from build123d import *
from build123d.topology import SkipClean

# Parameters (mm, degrees)
BOSS_EXTRUDE1_DEPTH      = 3.81
BOSS_EXTRUDE1_DEPTH_BACK = 6.35
SKETCH1_R                = 49.4538
SKETCH2_R                = 49.4538
BOSS_EXTRUDE2_DEPTH      = 381
SHELL1_T                 = -3.175
CUT_EXTRUDE1_DEPTH       = 398.363186857
BOSS_EXTRUDE3_DEPTH      = 3.81
SKETCH7_R                = 49.4538
SKETCH7_R_2              = 45.085
CUT_EXTRUDE2_DEPTH       = 6.35
BOSS_EXTRUDE4_START      = 7.62
BOSS_EXTRUDE4_DEPTH      = 7.62
SKETCH10_R               = 35.56
CUT_EXTRUDE3_DEPTH       = 6.35
SKETCH11_R               = 8.382
CUT_EXTRUDE4_DEPTH       = 5.08
SKETCH12_R               = 6.0325
CUT_EXTRUDE5_DEPTH       = 402.739558289
BOSS_EXTRUDE5_DEPTH      = 5.08
SKETCH14_R               = 4.191
CUT_EXTRUDE6_DEPTH       = 405.866453376
BOSS_EXTRUDE6_START      = 6.35
SKETCH15_R               = 4.191
SKETCH15_R_2             = 6.0325
BOSS_EXTRUDE6_DEPTH      = 6.35


with BuildPart() as part:
    # Sketch1 → Boss-Extrude1 (new, two sides: drawn at the far end of the back side and taken through both)
    with BuildSketch(Plane(origin=(0, 0, 0), x_dir=(1, 0, 0), z_dir=(0, 1, 0)).offset(-BOSS_EXTRUDE1_DEPTH_BACK)):
        with Locations(Location((0, 0, 0), (0, 0, 270))):
            Circle(SKETCH1_R)
    extrude(amount=BOSS_EXTRUDE1_DEPTH + BOSS_EXTRUDE1_DEPTH_BACK)

    # Sketch2 → Boss-Extrude2 (add)
    with BuildSketch(Plane(origin=(0, 3.81, 0), x_dir=(1, 0, 0), z_dir=(0, 1, 0))):
        with Locations(Location((0, 0, 0), (0, 0, 270))):
            Circle(SKETCH2_R)
    extrude(amount=BOSS_EXTRUDE2_DEPTH)

    # Shell1
    shell1_openings = [part.faces().sort_by_distance(p)[0] for p in [
        (0, 384.81, 0),
    ]]
    offset(amount=SHELL1_T, openings=shell1_openings, kind=Kind.INTERSECTION)

    # Sketch4 → Cut-Extrude1 (cut, through all)
    with BuildSketch(Plane.XZ.offset(6.35)):
        with BuildLine():
            Line((49.4538, 0), (12.7, 0))
            ThreePointArc((12.7, 0), (0, -12.7), (-12.7, 0))
            Line((-12.7, 0), (-49.4538, 0))
            ThreePointArc((-49.4538, 0), (0, -49.4538), (49.4538, 0))
        make_face()
    extrude(amount=-CUT_EXTRUDE1_DEPTH, mode=Mode.SUBTRACT)

    # Sketch5 → Boss-Extrude3 (add)
    with BuildSketch(Plane(origin=(0, -3.175, 0), x_dir=(1, 0, 0), z_dir=(0, 1, 0))):
        with BuildLine():
            Line((-46.2788, 0), (-12.7, 0))
            ThreePointArc((-12.7, 0), (0, 12.7), (12.7, 0))
            Line((12.7, 0), (46.2788, 0))
            ThreePointArc((46.2788, 0), (0, -46.2788), (-46.2788, 0))
        make_face()
    extrude(amount=BOSS_EXTRUDE3_DEPTH)

    # Sketch7 → Cut-Extrude2 (cut)
    with BuildSketch(Plane.XZ.offset(6.35)):
        Circle(SKETCH7_R)
        Circle(SKETCH7_R_2, mode=Mode.SUBTRACT)
    extrude(amount=-CUT_EXTRUDE2_DEPTH, mode=Mode.SUBTRACT)

    # Sketch9 → Boss-Extrude4 (add)
    with SkipClean():  # the faces are left unmerged after this step: merging them gives an invalid solid
        with BuildSketch(Plane.XZ.offset(6.35).offset(BOSS_EXTRUDE4_START)):
            with BuildLine():
                Line((45.085, 0), (12.7, 0))
                ThreePointArc((12.7, 0), (0, -12.7), (-12.7, 0))
                Line((-12.7, 0), (-45.085, 0))
                ThreePointArc((-45.085, 0), (0, 45.085), (45.085, 0))
            make_face()
        extrude(amount=-BOSS_EXTRUDE4_DEPTH)
    add(part.part.scale(1), mode=Mode.REPLACE)  # the faces are merged on a copy

    # Sketch10 → Cut-Extrude3 (cut)
    with BuildSketch(Plane(origin=(0, 0.635, 0), x_dir=(1, 0, 0), z_dir=(0, 1, 0))):
        Circle(SKETCH10_R)
    extrude(amount=-CUT_EXTRUDE3_DEPTH, mode=Mode.SUBTRACT)

    # Sketch11 → Cut-Extrude4 (cut)
    with BuildSketch(Plane(origin=(0, -5.715, 0), x_dir=(1, 0, 0), z_dir=(0, 1, 0))):
        with Locations(Location((0, 0, 0), (0, 0, 270))):
            Circle(SKETCH11_R)
    cut_extrude4 = extrude(amount=-CUT_EXTRUDE4_DEPTH, mode=Mode.SUBTRACT)

    # Sketch12 → Cut-Extrude5 (cut, through all)
    with BuildSketch(Plane(origin=(0, -10.795, 0), x_dir=(1, 0, 0), z_dir=(0, 1, 0))):
        with Locations(Location((0, 0, 0), (0, 0, 270))):
            Circle(SKETCH12_R)
    extrude(amount=-CUT_EXTRUDE5_DEPTH, mode=Mode.SUBTRACT)

    # Sketch13 → Boss-Extrude5 (add)
    with SkipClean():  # the faces are left unmerged after this step: merging them gives an invalid solid
        with BuildSketch(Plane(origin=(0, 0.635, 0), x_dir=(1, 0, 0), z_dir=(0, 1, 0))):
            with BuildLine():
                Line((-46.2788, 0), (-35.56, 0))
                ThreePointArc((-35.56, 0), (0, -35.56), (35.56, 0))
                Line((35.56, 0), (46.2788, 0))
                ThreePointArc((46.2788, 0), (0, -46.2788), (-46.2788, 0))
            make_face()
        extrude(amount=BOSS_EXTRUDE5_DEPTH)
    add(part.part.scale(1), mode=Mode.REPLACE)  # the faces are merged on a copy

    # Sketch14 → Cut-Extrude6 (cut, through all)
    with BuildSketch(Plane.XZ.offset(13.97)):
        with Locations(Location((0, 15.24, 0), (0, 0, 270))):
            Circle(SKETCH14_R)
    extrude(amount=-CUT_EXTRUDE6_DEPTH, mode=Mode.SUBTRACT)

    # Sketch15 → Boss-Extrude6 (add)
    with BuildSketch(Plane.XZ.offset(13.97).offset(BOSS_EXTRUDE6_START)):
        with BuildLine():
            Line((12.7, 0), (45.085, 0))
            ThreePointArc((45.085, 0), (0, 45.085), (-45.085, 0))
            Line((-45.085, 0), (-12.7, 0))
            ThreePointArc((-12.7, 0), (0, -12.7), (12.7, 0))
        make_face()
        with Locations(Location((0, 15.24, 0), (0, 0, 270))):
            Circle(SKETCH15_R, mode=Mode.SUBTRACT)
        with Locations(Location((0, 0, 0), (0, 0, 90))):
            Circle(SKETCH15_R_2, mode=Mode.SUBTRACT)
    extrude(amount=-BOSS_EXTRUDE6_DEPTH)

    # Mirror2: Cut-Extrude4 across plane
    add(cut_extrude4.mirror(Plane(origin=(0, -13.0175, 0), x_dir=(0, 0, 1), z_dir=(0, -1, 0))), mode=Mode.SUBTRACT)


solid = part.part
Geometry check sheet. Reference: the model listing, model coordinates, mm. A direction names the side the tool comes from. Give positions to 0.01 mm unless a question says otherwise; leave off trailing zeros. Loops run counter-clockwise (first coordinate to the right, second up) from the corner with the lowest first, then second, coordinate; pieces in that order, holes last. Notation, with made-up numbers: (45, 52.25) -> (60, 52.25) arc R25 cw to (60, 83.25) -> close; hole circle Ø4 at (10.5, 76.5). An arc over 180 degrees is marked (long way). Answer in a Markdown table with one row per item. Add a question column.
1) Cross-section at A-A on z = 15.24. Record the boundary of the cut face in (x, y) (3 decimals).
2) Draft check along X on faces 1 (the face through (-5.1, -8.22, -6.65)), 2 (the face through (0, 384.81, 47)), 3 (the face through (0.991, -10.302, 45.074)). Enter one of: pulls with the +X half, pulls with the -X half, needs draft (parallel to the pull), parting line crosses it, or undercut.
3) Cross-section at D-D on x = 20. Record the boundary of the cut face in (y, z) (3 decimals).
4) Material ranges on probe 1 along Y at (x, z) = (-37, 28.5); probe 2 along Y at (x, z) = (-21, 11) (3 decimals); probe 3 along Z at (x, y) = (2.5, 214), recorded low to high. Write a range as from..to.
5) Gauge pin test, flat ends, axial feed: P1, Ø12, axis at y = 183.5, z = 31.5, coming from the +X side; P2, Ø12, axis at y = 244, z = 8, coming from the -X side; P3, Ø5, axis at x = 0, z = 15.24, coming from the +Y side; P4, Ø4, axis at x = -36.5, y = 174, coming from the -Z side. Record the tip position at first contact, or that the pin passes through.
6) Set-up check for faces 4 (the face through (47, 106, 0)), 5 (the face through (6, -10.795, -2)), 6 (the face through (6, -15.24, -2)), 7 (the face through (7, -5.715, 11)): record each of +Z, -Z, +X, -X, +Y, -Y from which the full face is reachable in a straight line by a thin tool's end or side.
7) Cross-section at C-C on y = 162. Record the boundary of the cut face in (x, z).
8) Cross-section at B-B on x = 0. Record the boundary of the cut face in (y, z) (1 decimal), and give its area (3 significant figures).
Outcome:
| question | item | result |
|---|---|---|
| 1 | outline | (-47.047, 0) -> (-42.431, 0) -> (-42.431, -20.32) -> (-4.191, -20.32) -> (-4.191, -5.715) -> (-32.129, -5.715) -> (-32.129, 5.715) -> (-43.697, 5.715) -> (-43.697, 384.81) -> (-47.047, 384.81) -> close; (4.191, -20.32) -> (42.431, -20.32) -> (42.431, 0) -> (47.047, 0) -> (47.047, 384.81) -> (43.697, 384.81) -> (43.697, 5.715) -> (32.129, 5.715) -> (32.129, -5.715) -> (4.191, -5.715) -> close |
| 2 | face 1 | undercut |
| 2 | face 2 | needs draft |
| 2 | face 3 | parting line crosses it |
| 3 | outline | (-20.32, 0) -> (-5.715, 0) -> (-5.715, 29.403) -> (5.715, 29.403) -> (5.715, 41.734) -> (384.81, 41.734) -> (384.81, 45.229) -> (0, 45.229) -> (0, 40.406) -> (-20.32, 40.406) -> close |
| 4 | probe 1 | y = 0..384.81 |
| 4 | probe 2 | y = -20.32..-5.715 |
| 4 | probe 3 | z = 46.21..49.39 |
| 5 | P1 | stops at x = 42.37 |
| 5 | P2 | stops at x = -49.41 |
| 5 | P3 | passes through |
| 5 | P4 | stops at z = 25.68 |
| 6 | face 4 | -Z, +X, +Y, -Y |
| 6 | face 5 | +Y |
| 6 | face 6 | -Y |
| 6 | face 7 | -Z, +Y |
| 7 | outline | (-49.45, 0) -> (-46.28, 0) arc R46.28 cw to (46.28, 0) -> (49.45, 0) arc R49.45 ccw to start |
| 8 | outline | (-20.3, -12.7) -> (-5.7, -12.7) -> (-5.7, -8.4) -> (-10.8, -8.4) -> (-10.8, -6) -> (-15.2, -6) -> (-15.2, -8.4) -> (-20.3, -8.4) -> close; (-20.3, 8.4) -> (-15.2, 8.4) -> (-15.2, 6) -> (-10.8, 6) -> (-10.8, 8.4) -> (-5.7, 8.4) -> (-5.7, 11) -> (-20.3, 11) -> close; (-20.3, 19.4) -> (-5.7, 19.4) -> (-5.7, 35.6) -> (5.7, 35.6) -> (5.7, 46.3) -> (384.8, 46.3) -> (384.8, 49.5) -> (0, 49.5) -> (0, 45.1) -> (-20.3, 45.1) -> close |
| 8 | area | 1,840 mm^2 |
